Autodesk Inventor part; units mm, degrees
ref_plane "YZ Plane" through (0, 0, 0) normal (1, 0, 0) x (0, 1, 0)
ref_plane "XZ Plane" through (0, 0, 0) normal (0, 1, 0) x (-1, 0, 0)
ref_plane "XY Plane" through (0, 0, 0) normal (0, 0, 1) x (1, 0, 0)
sketch "Sketch1" plane through (0, 0, 0) normal (0, 0, 1) x (1, 0, 0)
  line L0 (0, 0) -> (-5, 0)
  line L1 (0, 0) -> (5, 0)
  line L2 (-5, 0) -> (-5, -4) construction
  line L3 (-5, -4) -> (-23.8125, -4) construction
  line L4 (-5, 0) -> (10, 0) construction
  line L5 (0, -6.9282) -> (-35, -6.9282) construction
  line L6 (-12.5, -12.9904) -> (-35, -12.9904)
  line L7 (-23.8125, -4) -> (-23.8125, -8) construction
  line L8 (-35, -12.9904) -> (-35, -8)
  line L9 (-35, 0) -> (-35, 6)
  line L10 (-35, 6) -> (0, 6)
  line L11 (0, 6) -> (0, 0) construction
  line L12 (0, 0) -> (5, 0)
  line L13 (12.5, -12.9904) -> (35, -12.9904)
  line L14 (35, -12.9904) -> (35, -8)
  line L15 (35, 0) -> (35, 6)
  line L16 (35, 6) -> (0, 6)
  line L17 (-5, 0) -> (-5, -5)
  line L18 (-5, -5) -> (-12.5, -12.9904)
  line L19 (5, 0) -> (5, -5)
  line L20 (5, -5) -> (12.5, -12.9904)
  line L21 (-25, 0) -> (-21, 0)
  line L22 (-35, 0) -> (-35, -8)
  line L23 (35, 0) -> (35, -8)
  dimension "d0" = 5
  dimension "d1" = 5
  dimension "d2" = 4
  dimension "d3" = 15
  dimension "d5" = 35
  dimension "d10" = 6
  dimension "d24" = 5
  dimension "d25" = 5
  dimension "d27" = 4
extrude "Extrusion1" add sketch "Sketch1" along normal mid plane 15
sketch "Sketch5" plane through (-35, 6, 7.5) normal (0, 1, 0) x (1, 0, 0)
  circle A0 centre (35, 7.5) radius 2 construction
  line L0 (35, 7.5) -> (35, 13.5) construction
  line L1 (35, 7.5) -> (25, 7.5) construction
  line L2 (35, 13.5) -> (25, 13.5)
  line L3 (25, 13.5) -> (25, 1.5)
  line L4 (25, 1.5) -> (45, 1.5)
  line L5 (45, 1.5) -> (45, 13.5)
  line L6 (45, 13.5) -> (35, 13.5)
  line L7 (25, 13.5) -> (25, 15)
  line L8 (0, 15) -> (70, 15)
  line L9 (45, 13.5) -> (45, 15)
  line L10 (45, 15) -> (25, 15)
  line L11 (25, 1.5) -> (25, 0)
  line L12 (25, 0) -> (45, 0)
  line L13 (40, 0) -> (47.5, 0)
  line L14 (45, 1.5) -> (45, 0)
  dimension "d40" = 6
  dimension "d41" = 10
  dimension "d42" = 12
  dimension "d43" = 20
  dimension "d44" = 12
extrude "Extrusion5" cut sketch "Sketch5" against normal blind 18 contours L2 L7 L8 L9 L6 | L4 L14 L12 L11
sketch "Sketch6" plane through (35, 6, 7.5) normal (0, 1, 0) x (1, 0, 0)
  circle A0 centre (-35, 7.5) radius 4
  dimension "d47" = 8
extrude "Extrusion6" cut sketch "Sketch6" against normal blind 6
sketch "Sketch7" plane through (35, 6, 7.5) normal (0, 1, 0) x (1, 0, 0)
  line L0 (-35, 7.5) -> (-65, 7.5) construction
  line L1 (-65, 7.5) -> (-65, 11.5) construction
  line L2 (-65, 11.5) -> (-65, 3.5) construction
  line L3 (-65, 3.5) -> (-70, 3.5)
  line L4 (-70, 15) -> (-70, 0)
  line L5 (-70, 3.5) -> (-70, 11.5)
  line L6 (-70, 11.5) -> (-65, 11.5)
  line L7 (-70, 11.5) -> (-65, 11.5)
  line L8 (-70, 11.5) -> (-56, 11.5)
  line L9 (-56, 11.5) -> (-56, 3.5)
  line L10 (-56, 3.5) -> (-70, 3.5)
  circle A0 centre (-35, 7.5) radius 4 construction
  line L11 (-35, 7.5) -> (-35, 1.5875) construction
  line L12 (0, 15) -> (0, 0)
  line L13 (0, 11.5) -> (-14, 11.5)
  line L14 (-14, 11.5) -> (-14, 3.5)
  line L15 (-14, 3.5) -> (0, 3.5)
  dimension "d50" = 30
  dimension "d51" = 4
  dimension "d52" = 8
  dimension "d53" = 14
extrude "Extrusion7" cut sketch "Sketch7" against normal blind 19
sketch "Sketch8" plane through (0, 0, 7.5) normal (0, 0, 1) x (1, 0, 0)
  line L0 (0, 0) -> (-30, 0) construction
  line L1 (-21, 6) -> (-35, 6) construction
  line L2 (-30, 6) -> (-30, -3.5) construction
  line L3 (-30, 6) -> (-20.5, 6) construction
  circle A0 centre (-30, -3.5) radius 3
  line L4 (0, 0) -> (0, -2.1213) construction
  circle A1 centre (30, -3.5) radius 3
  dimension "d56" = 30
  dimension "d57" = 9.5
  dimension "d58" = 90
  dimension "d59" = 6
extrude "Extrusion8" cut sketch "Sketch8" against normal blind 15
sketch "Sketch9" plane through (-35, -12.9904, -7.5) normal (0, -1, 0) x (1, 0, 0)
  line L0 (14, 3.5) -> (14, 11.5) construction
  line L1 (14, 11.5) -> (14, 11.5) construction
  line L2 (14, 11.5) -> (25.4, 11.5)
  line L3 (25.4, 11.5) -> (25.4, 3.5)
  line L4 (25.4, 3.5) -> (14, 3.5)
  line L5 (35, 7.5) -> (35, 13.3991) construction
  line L6 (14, 11.5) -> (14, 3.5)
  line L7 (56, 3.5) -> (56, 11.5) construction
  line L8 (56, 11.5) -> (44.6, 11.5)
  line L9 (44.6, 11.5) -> (44.6, 3.5)
  line L10 (44.6, 3.5) -> (56, 3.5)
  line L11 (56, 3.5) -> (56, 11.5)
  dimension "d62" = 0
  dimension "d63" = 90
  dimension "d64" = 8
extrude "Extrusion9" cut sketch "Sketch9" against normal blind 3
equation "\"BendRadius\" = Thickness"
equation "\"BendReliefWidth\" = Thickness"
equation "\"BendReliefDepth\" = 0.5 * Thickness"
equation "\"CornerReliefSize\" = 4 * Thickness"
equation "\"MinimumRemnant\" = 2 * Thickness"
equation "\"TransitionRadius\" = BendRadius"
equation "\"JacobiRadiusSize\" = BendRadius"
equation "\"GapSize\" = Thickness"
properties part number "Belka" material "Aluminum 6061"
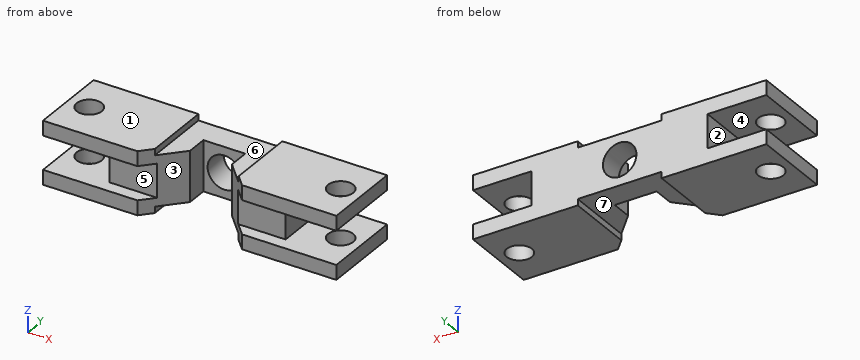
Can you work these out from the model? Positions are in its coordinate system, mm. Face numbers are marked on the shaded views. A direction names the side the tool comes from. Coordinates: 2 decimals unless noted, no trailing zeros. Write each loop counter-clockwise with the first axis right and the second up, starting at its lowest first coordinate (ties: lowest second). Pieces come first, ordered by that corner, then holes. Notation, with made-up numbers: (9, 4) -> (63, 4) arc R14 cw to (63, 11) -> close; hole circle Ø3 at (79.25, 68). An arc over 180 degrees is marked (long way). Write item = value, one per line.
(1) Imagine slicing it at B-B (x = -30). Please give me the cut outline in (y, z).
Verdict:
outline = (-12.99, -7.5) -> (-6.5, -7.5) -> (-6.5, -4) -> (-12.99, -4) -> close; (-12.99, 4) -> (-6.5, 4) -> (-6.5, 7.5) -> (-12.99, 7.5) -> close; (-0.5, -7.5) -> (6, -7.5) -> (6, -4) -> (-0.5, -4) -> close; (-0.5, 4) -> (6, 4) -> (6, 7.5) -> (-0.5, 7.5) -> close
(2) If I drill on probe 1 along X at (y, z) = (4.6, 0); probe 2 along Z at (x, y) = (-21.5, -4.75); probe 3 along Y at (x, z) = (-30, -5.7), over which ranges is the centre line in solid material (lowest first)?
Verdict:
probe_1 = -21 to -4, 4 to 21
probe_2 = -7.5 to -4, 4 to 7.5
probe_3 = -12.99 to -6.5, -0.5 to 6
(3) Imagine slicing it at A-A (z = 0). Please give me the cut outline in (x, y), and give its area (3 significant figures).
Verdict:
outline = (-21, -9.99) -> (-9.68, -9.99) -> (-5, -5) -> (-5, 0) -> (-4, 0) -> (-4, 6) -> (-21, 6) -> close; (4, 0) -> (5, 0) -> (5, -5) -> (9.68, -9.99) -> (21, -9.99) -> (21, 6) -> (4, 6) -> close
area = 500 mm^2
(4) Imagine slicing it at C-C (y = -8). Please give me the cut outline in (x, z).
Verdict:
outline = (-35, -7.5) -> (-10, -7.5) -> (-10, -6) -> (-7.82, -6) -> (-7.82, 6) -> (-10, 6) -> (-10, 7.5) -> (-35, 7.5) -> (-35, 4) -> (-21, 4) -> (-21, -4) -> (-35, -4) -> close; (7.82, -6) -> (10, -6) -> (10, -7.5) -> (35, -7.5) -> (35, -4) -> (21, -4) -> (21, 4) -> (35, 4) -> (35, 7.5) -> (10, 7.5) -> (10, 6) -> (7.82, 6) -> close
(5) Imagine slicing it at D-D (z = 5). Please give me the cut outline in (x, y), and give its area (3 significant figures).
Verdict:
outline = (-35, -12.99) -> (-12.5, -12.99) -> (-5, -5) -> (-5, 0) -> (5, 0) -> (5, -5) -> (12.5, -12.99) -> (35, -12.99) -> (35, 6) -> (-35, 6) -> close; hole circle Ø6 at (-30, -3.5); hole circle Ø6 at (30, -3.5)
area = 1,080 mm^2
(6) On a 3-axis mill with a long thin cutter (end or side, diameter ignored), from which of +Z, -Z, +X, -X, +Y, -Y can I reach the whole of each face in a straight line? I mean the marked faces 5, 6 and 7. Say none if no direction works.
Verdict:
face_5 = +X, -X, -Y
face_6 = +Z, +Y, -Y
face_7 = -Z, +Y, -Y
(7) For pin 1 (1.5 mm diameter, centred on y = -3.5, z = -1.5, fed in from -X); pin 2 (8 mm diameter, centred on x = 3.5, y = -2.5, fed in from -Z); pin 3 (2.5 mm diameter, centred on y = -2, z = -1, fed in from +X); pin 4 (3.5 mm diameter, centred on x = 30, y = -3.5, fed in from -Z), each with a flat end and sliding along its axis, tell me the tip position at first contact or that it passes through.
Verdict:
pin_1 = -21
pin_2 = -6
pin_3 = 21
pin_4 = through
(8) Thinking about a two-plate mould opening in Z: for the marked faces 1, 2, 3 and 4, which applies, +Z half, -Z half, draft (parallel to the pull), parting line (faces both ways), or undercut?
Verdict:
face_1 = +Z half
face_2 = undercut
face_3 = draft
face_4 = undercut
